```python
from build123d import *

# Parameters (mm, degrees)
F0_W     = 3
F0_H     = 10
F1_DEPTH = 1
F2_W     = 1
F2_H     = 10
F5_D     = 4.3
F5_DEPTH = 2.5


with BuildPart() as f1:
    # F0 (on Front) → F1 (new body)
    with BuildSketch(Plane.XZ):
        Polygon((5, 10), (5, 20), (-5, 20), (-5, -20), (5, -20), (5, -10), align=None)
        with Locations((6.5, -15)):
            Rectangle(F0_W, F0_H)
        with Locations((6.5, 15)):
            Rectangle(F0_W, F0_H)
    extrude(amount=F1_DEPTH)

    # F2 (on face) → F3 (revolve)
    with BuildSketch(Plane.YZ.offset(8)):
        with Locations((-0.5, -15)):
            Rectangle(F2_W, F2_H)
        with Locations((-0.5, 15)):
            Rectangle(F2_W, F2_H)
    revolve(axis=Axis((8, 1, 0), (0, 0, 1)))

    # F5
    with Locations(Plane.XZ.offset(1)):
        with Locations((0, 13), (0, -13)):
            Hole(F5_D / 2, depth=F5_DEPTH)


solid = f1.part
```
Source: CAD feature listing. Evaluate the final solid. Frame: model axes, mm. A direction names the side the tool comes from. Round coordinates to 2 decimals unless told otherwise and drop trailing zeros. Loops run counter-clockwise (first coordinate to the right, second up) from the corner with the lowest first, then second, coordinate; pieces in that order, holes last. Notation, with made-up numbers: M -15.5,-36 L 3.5,-36 A33 cw 3.5,2 Z; hole C 88.25,86.5 d6. An arc over 180 degrees is marked long. Use a Markdown table: item, result. Add a question column.
1. Contact query for flat-ended pins moving along their axis: pin 1 (4 mm diameter, centred on x = 0.5, z = -9.5, fed in from +Y); pin 2 (1.8 mm diameter, centred on x = 8, y = 1, fed in from -Z). Output: stop coordinate, or through.
2. Cut plane D-D, the plane z = 1.5. Output: boundary loops of the cut face in (x, y).
3. Cut plane A-A, the plane z = 13. Output: boundary loops of the cut face in (x, y), and give its area (3 significant figures).
4. Ray query, line 1 along Z through (x, y) = (0, -0.4); line 2 along X through (y, z) = (1, -12.5); line 3 along Y through (x, z) = (-3.75, 17.5). Return the intervals inside material, ascending. Write a range as [from, to].
5. Cut plane B-B, the plane x = 0. Output: boundary loops of the cut face in (y, z), and give its area (3 significant figures).
6. Pull-direction query (Z, two-part tool) for faces 3 (the flat face through (-5, -0.5, 0.3)), 4 (the flat face through (3.6, -0.2, -20)), 5 (the flat face through (5, -0.5, -0.1)); classes: +Z half, -Z half, draft (parallel to the pull), parting line (faces both ways), or undercut.
7. Set-up query: faces 1 (the cylindrical face through (-0.99, -0.49, -14.91)), 2 (the flat face through (7, 0, 10)). Return all of +Z, -Z, +X, -X, +Y, -Y with unobstructed straight access to the full face (end or side cutting, diameter ignored); none if empty.
8. Cut plane C-C, the plane y = 1. Output: boundary loops of the cut face in (x, z), and give its area (3 significant figures).
Solution:
| question | item | result |
|---|---|---|
| 1 | pin 1 | stops at y = 0 |
| 1 | pin 2 | passes through |
| 2 | outline | M -5,-1 L 5,-1 L 5,0 L -5,0 Z |
| 3 | outline | M -5,-1 L -2.15,-1 L -2.15,0 L -5,0 Z; M 2.15,-1 L 8,-1 A2 ccw long 6.27,0 L 2.15,0 Z; hole C 8,1 d2 |
| 3 | area | 16.9 mm2 |
| 4 | line 1 | z = [-20, -15.15], [-10.85, 10.85], [15.15, 20] |
| 4 | line 2 | x = [6, 7], [9, 10] |
| 4 | line 3 | y = [-1, 0] |
| 5 | outline | M -1,-20 L 0,-20 L 0,-15.15 L -1,-15.15 Z; M -1,-10.85 L 0,-10.85 L 0,10.85 L -1,10.85 Z; M -1,15.15 L 0,15.15 L 0,20 L -1,20 Z |
| 5 | area | 31.4 mm2 |
| 6 | face 3 | draft |
| 6 | face 4 | -Z half |
| 6 | face 5 | undercut |
| 7 | face 1 | +Y, -Y |
| 7 | face 2 | +X, +Y, -Y |
| 8 | outline | M 6,-20 L 7,-20 L 7,-10 L 6,-10 Z; M 6,10 L 7,10 L 7,20 L 6,20 Z; M 9,-20 L 10,-20 L 10,-10 L 9,-10 Z; M 9,10 L 10,10 L 10,20 L 9,20 Z |
| 8 | area | 40.0 mm2 |
